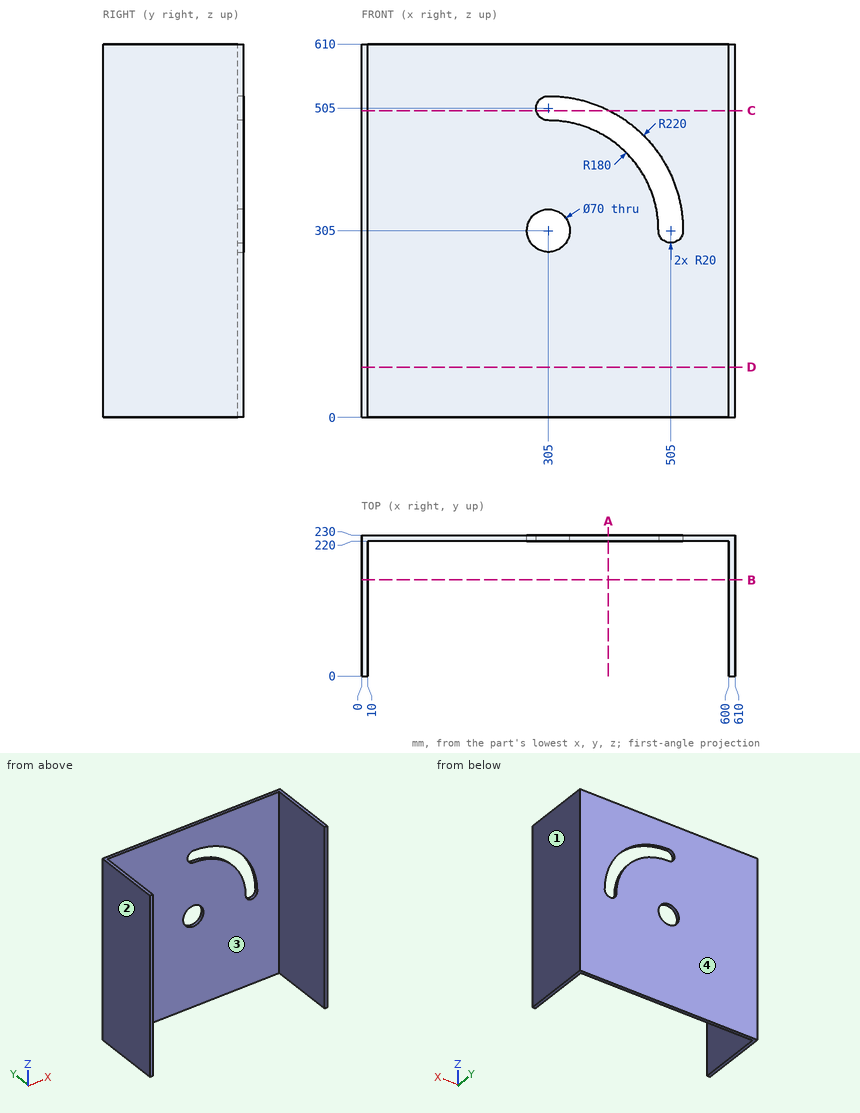
Study the drawing (mm; zero at the part's minimum x, y, z) and answer. Round coordinates to 2 decimals unless told otherwise and drop trailing zeros. Write each loop counter-clockwise with the first axis right and the second up, starting at its lowest first coordinate (ties: lowest second). Pieces come first, ordered by that corner, then holes. Notation, with made-up numbers: (85.25, 30.25) -> (117.25, 30.25) arc R13 ccw to (117.25, 53.25) -> close; hole circle Ø1 at (87.25, -38). An arc over 180 degrees is marked (long way). Use CSV: the item, a comma, the result in double quotes. Start each with the question number.
(1) Section C-C on z = 501 is taken. Give the vertices of the cut face in (x, y), then the cut area to 3 significant figures.
(2) Section B-B on y = 157 is taken. Give the vertices of the cut face in (x, z), then the cut area to 3 significant figures.
(3) Each of these flat-tipped pins is pushed along its axis until it touches: pin 1 (1.5 mm diameter, centred on y = 39.5, z = 456, fed in from -X); pin 2 (3 mm diameter, centred on x = 141.5, z = 415, fed in from -Y). Where does it stop, or does it pass through?
(4) The mould has two halves that part along X. Classify the marked faces 1, 2, 3 and 4: released by +X, released by -X, zero draft, split by the parting line, or undercut.
(5) Section D-D on z = 82 is taken. Give the vertices of the cut face in (x, y), then the cut area to 3 significant figures.
(6) Consider L1, parallel to X at y = 222.5, z = 305; L2, parallel to X at y = 214, z = 56; L3, parallel to Y at x = 184.5, z = 74.5. Determine where each line is inside the solid, lowest interval first. Write a range as from..to.
(7) Section A-A on x = 403 is taken. Give the vertices of the cut face in (y, z).
A:
1,outline,"(0, 0) -> (10, 0) -> (10, 220) -> (285.4, 220) -> (285.4, 230) -> (0, 230) -> close; (404.92, 220) -> (600, 220) -> (600, 0) -> (610, 0) -> (610, 230) -> (404.92, 230) -> close"
1,area,"9,300 mm²"
2,outline,"(0, 0) -> (10, 0) -> (10, 610) -> (0, 610) -> close; (600, 0) -> (610, 0) -> (610, 610) -> (600, 610) -> close"
2,area,"12,200 mm²"
3,pin 1,"stops at x = 0"
3,pin 2,"stops at y = 220"
4,face 1,"released by +X"
4,face 2,"released by -X"
4,face 3,"undercut"
4,face 4,"zero draft"
5,outline,"(0, 0) -> (10, 0) -> (10, 220) -> (600, 220) -> (600, 0) -> (610, 0) -> (610, 230) -> (0, 230) -> close"
5,area,"10,500 mm²"
6,L1,"x = 0..270, 340..485, 525..610"
6,L2,"x = 0..10, 600..610"
6,L3,"y = 220..230"
7,outline,"(220, 0) -> (230, 0) -> (230, 455.98) -> (220, 455.98) -> close; (220, 501.97) -> (230, 501.97) -> (230, 610) -> (220, 610) -> close"
